Input: part model. Units: mm. Frame: model coordinates. A direction names the side the tool comes from. Coordinates: 2 decimals unless noted, no trailing zeros. Write each loop counter-clockwise with the first axis right and the second up, starting at its lowest first coordinate (ties: lowest second). Pieces come first, ordered by that corner, then holes. Notation, with made-up numbers: M 45,59 L 67,59 A29 ccw 67,85 Z; hole C 24,0 d2. An arc over 180 degrees is marked long. Write each question's results on one line, items separated by ' | '. Start each with the question number.
1. First-contact query: pin 1 (1 mm diameter, centred on y = 86, z = 6.5, fed in from -X); pin 2 (2 mm diameter, centred on x = -41.5, z = 8, fed in from +Y); pin 3 (1 mm diameter, centred on y = 25, z = 4.5, fed in from +X). Flat tips, straight axial feed; report the tip coordinate or a pass-through.
2. Section query B-B, the plane x = -20.5. Output: boundary loops of the cut face in (y, z) (3 decimals).
3. Section query C-C, the plane y = 9. Output: boundary loops of the cut face in (x, z).
4. Section query A-A, the plane z = 4.75. Output: boundary loops of the cut face in (x, y).
5. Set-up query: faces 1 (the flat face through (-98, 98, 2.54)), 2 (the flat face through (-94, 99, 10.16)), 3 (the flat face through (-139, 0, 2)). Return all of +Z, -Z, +X, -X, +Y, -Y with unobstructed straight access to the full face (end or side cutting, diameter ignored); none if empty.
6. Pull-direction query (X, two-part tool) for faces 4 (the flat face through (0, 137, 4)), 5 (the flat face through (-89, 89, 0)), 6 (the cylindrical face through (-4.45, 4.53, 1.25)); classes: +X half, -X half, draft (parallel to the pull), parting line (faces both ways), or undercut.
7. Ray query, probe 1 along Z at (x, y) = (-120.5, 67); probe 2 along Y at (x, z) = (-57.15, 1.3); probe 3 along X at (y, z) = (64.5, 3.75). Return the intervals inside material, ascending.
8. Section query D-D, the plane x = -63.5. Output: boundary loops of the cut face in (y, z), and give its area (3 significant figures).
```python
from build123d import *

# Parameters (mm, degrees)
F1_DEPTH = 2.54
F2_DEPTH = 7.62
F3_DEPTH = 2.54
F4_DEPTH = 15.24


with BuildPart() as f1:
    # F0 (on Top) → F1 (new body)
    with BuildSketch(Plane.XY):
        with BuildLine():
            Line((-6.2754395375, 0.9702363687), (-12.7, 1.9635281017))
            Line((-12.7, 1.9635281017), (-12.7, 0))
            Line((-12.7, 0), (-6.35, 0))
            ThreePointArc((-6.35, 0), (-6.3313324452, 0.4865485263), (-6.2754395375, 0.9702363687))
        make_face()
        with BuildLine():
            Line((-6.35, 0), (-2.54, 0))
            ThreePointArc((-2.54, 0), (-2.5325329781, 0.1946194105), (-2.510175815, 0.3880945475))
            Line((-2.510175815, 0.3880945475), (-6.2754395375, 0.9702363687))
            ThreePointArc((-6.2754395375, 0.9702363687), (-6.3313324452, 0.4865485263), (-6.35, 0))
        make_face()
        with BuildLine():
            ThreePointArc((-2.510175815, 0.3880945475), (-1.7960512242, 1.7960512242), (-0.3880945475, 2.510175815))
            Line((-0.3880945475, 2.510175815), (-0.9702363687, 6.2754395375))
            ThreePointArc((-0.9702363687, 6.2754395375), (-4.4901280605, 4.4901280605), (-6.2754395375, 0.9702363687))
            Line((-6.2754395375, 0.9702363687), (-2.510175815, 0.3880945475))
        make_face()
        with BuildLine():
            Line((0, 2.54), (0, 6.35))
            ThreePointArc((0, 6.35), (-0.4865485263, 6.3313324452), (-0.9702363687, 6.2754395375))
            Line((-0.9702363687, 6.2754395375), (-0.3880945475, 2.510175815))
            ThreePointArc((-0.3880945475, 2.510175815), (-0.1946194105, 2.5325329781), (0, 2.54))
        make_face()
        with BuildLine():
            Line((0, 6.35), (0, 12.7))
            Line((0, 12.7), (-1.9635281017, 12.7))
            Line((-1.9635281017, 12.7), (-0.9702363687, 6.2754395375))
            ThreePointArc((-0.9702363687, 6.2754395375), (-0.4865485263, 6.3313324452), (0, 6.35))
        make_face()
        with BuildLine():
            Line((0, 12.7), (0, 30.48))
            ThreePointArc((0, 30.48), (-2.3354329262, 30.3903957369), (-4.6571345698, 30.12210978))
            Line((-4.6571345698, 30.12210978), (-1.9635281017, 12.7))
            Line((-1.9635281017, 12.7), (0, 12.7))
        make_face()
        with BuildLine():
            Line((-12.7, 1.9635281017), (-30.12210978, 4.6571345698))
            ThreePointArc((-30.12210978, 4.6571345698), (-30.3903957369, 2.3354329262), (-30.48, 0))
            Line((-30.48, 0), (-12.7, 0))
            Line((-12.7, 0), (-12.7, 1.9635281017))
        make_face()
        with BuildLine():
            Line((-30.12210978, 4.6571345698), (-82.1429547439, 12.7))
            ThreePointArc((-82.1429547439, 12.7), (-79.6054840123, 6.5740037456), (-78.74, 0))
            Line((-78.74, 0), (-30.48, 0))
            ThreePointArc((-30.48, 0), (-30.3903957369, 2.3354329262), (-30.12210978, 4.6571345698))
        make_face()
        with BuildLine():
            Line((-12.7, 126.1370452561), (-12.7, 134.0196045361))
            ThreePointArc((-12.7, 134.0196045361), (-95.1907148833, 95.1907148833), (-134.0196045361, 12.7))
            Line((-134.0196045361, 12.7), (-126.1370452561, 12.7))
            ThreePointArc((-126.1370452561, 12.7), (-104.14, 25.4), (-82.1429547439, 12.7))
            Line((-82.1429547439, 12.7), (-57.15, 12.7))
            ThreePointArc((-57.15, 12.7), (-88.5808964237, 88.5808964237), (-12.7, 57.15))
            Line((-12.7, 57.15), (-12.7, 82.1429547439))
            ThreePointArc((-12.7, 82.1429547439), (-25.4, 104.14), (-12.7, 126.1370452561))
        make_face()
        with BuildLine():
            Line((-126.1370452561, 12.7), (-134.0196045361, 12.7))
            ThreePointArc((-134.0196045361, 12.7), (-134.4698173618, 6.3570919986), (-134.62, 0))
            Line((-134.62, 0), (-129.54, 0))
            ThreePointArc((-129.54, 0), (-128.6745159877, 6.5740037456), (-126.1370452561, 12.7))
        make_face()
        with BuildLine():
            Line((-57.15, 12.7), (-82.1429547439, 12.7))
            Line((-82.1429547439, 12.7), (-30.12210978, 4.6571345698))
            ThreePointArc((-30.12210978, 4.6571345698), (-29.1934246673, 8.7620977053), (-27.7081287712, 12.7))
            Line((-27.7081287712, 12.7), (-57.15, 12.7))
        make_face()
        with BuildLine():
            Line((-12.7, 27.7081287712), (-12.7, 57.15))
            ThreePointArc((-12.7, 57.15), (-25.7191035763, 25.7191035763), (-57.15, 12.7))
            Line((-57.15, 12.7), (-27.7081287712, 12.7))
            ThreePointArc((-27.7081287712, 12.7), (-21.5526146906, 21.5526146906), (-12.7, 27.7081287712))
        make_face()
        with BuildLine():
            Line((-4.6571345698, 30.12210978), (-12.7, 82.1429547439))
            Line((-12.7, 82.1429547439), (-12.7, 57.15))
            Line((-12.7, 57.15), (-12.7, 27.7081287712))
            ThreePointArc((-12.7, 27.7081287712), (-8.7620977053, 29.1934246673), (-4.6571345698, 30.12210978))
        make_face()
        with BuildLine():
            Line((0, 30.48), (0, 78.74))
            ThreePointArc((0, 78.74), (-6.5740037456, 79.6054840123), (-12.7, 82.1429547439))
            Line((-12.7, 82.1429547439), (-4.6571345698, 30.12210978))
            ThreePointArc((-4.6571345698, 30.12210978), (-2.3354329262, 30.3903957369), (0, 30.48))
        make_face()
        with BuildLine():
            Line((0, 129.54), (0, 134.62))
            ThreePointArc((0, 134.62), (-6.3570919986, 134.4698173618), (-12.7, 134.0196045361))
            Line((-12.7, 134.0196045361), (-12.7, 126.1370452561))
            ThreePointArc((-12.7, 126.1370452561), (-6.5740037456, 128.6745159877), (0, 129.54))
        make_face()
    extrude(amount=F1_DEPTH)

    # F0 (on Top) → F2 (join)
    with BuildSketch(Plane.XY):
        with BuildLine():
            ThreePointArc((-134.62, 0), (-134.4698173618, 6.3570919986), (-134.0196045361, 12.7))
            Line((-134.0196045361, 12.7), (-136.5707713971, 12.7))
            ThreePointArc((-136.5707713971, 12.7), (-137.0126136617, 6.3568307817), (-137.16, 0))
            Line((-137.16, 0), (-134.62, 0))
        make_face()
        with BuildLine():
            ThreePointArc((-134.0196045361, 12.7), (-95.1907148833, 95.1907148833), (-12.7, 134.0196045361))
            Line((-12.7, 134.0196045361), (-12.7, 136.5707713971))
            ThreePointArc((-12.7, 136.5707713971), (-96.9867661075, 96.9867661075), (-136.5707713971, 12.7))
            Line((-136.5707713971, 12.7), (-134.0196045361, 12.7))
        make_face()
        with BuildLine():
            ThreePointArc((-12.7, 134.0196045361), (-6.3570919986, 134.4698173618), (0, 134.62))
            Line((0, 134.62), (0, 137.16))
            ThreePointArc((0, 137.16), (-6.3568307817, 137.0126136617), (-12.7, 136.5707713971))
            Line((-12.7, 136.5707713971), (-12.7, 134.0196045361))
        make_face()
    extrude(amount=F2_DEPTH)

    # F0 (on Top) + F2_face (on face) → F3 (join)
    with BuildSketch(Plane.XY):
        with BuildLine():
            ThreePointArc((-137.16, 0), (-137.0126136617, 6.3568307817), (-136.5707713971, 12.7))
            Line((-136.5707713971, 12.7), (-141.6719012366, 12.7))
            ThreePointArc((-141.6719012366, 12.7), (-142.0979043334, 6.3563499), (-142.24, 0))
            Line((-142.24, 0), (-137.16, 0))
        make_face()
        with BuildLine():
            ThreePointArc((-136.5707713971, 12.7), (-96.9867661075, 96.9867661075), (-12.7, 136.5707713971))
            Line((-12.7, 136.5707713971), (-12.7, 141.6719012366))
            ThreePointArc((-12.7, 141.6719012366), (-100.578868556, 100.578868556), (-141.6719012366, 12.7))
            Line((-141.6719012366, 12.7), (-136.5707713971, 12.7))
        make_face()
        with BuildLine():
            ThreePointArc((-12.7, 136.5707713971), (-6.3568307817, 137.0126136617), (0, 137.16))
            Line((0, 137.16), (0, 142.24))
            ThreePointArc((0, 142.24), (-6.3563499, 142.0979043334), (-12.7, 141.6719012366))
            Line((-12.7, 141.6719012366), (-12.7, 136.5707713971))
        make_face()
    with BuildSketch(Plane(origin=(-86.5127795808, 86.5127795808, 7.62), x_dir=(1, 0, 0), z_dir=(0, 0, 1))):
        with BuildLine():
            Line((-50.6472204192, -86.5127795808), (-48.1072204192, -86.5127795808))
            ThreePointArc((-48.1072204192, -86.5127795808), (-8.6779353026, 8.6779353025), (86.5127795808, 48.1072204192))
            Line((86.5127795808, 48.1072204192), (86.5127795808, 50.6472204192))
            ThreePointArc((86.5127795808, 50.6472204192), (-10.4739865268, 10.4739865267), (-50.6472204192, -86.5127795808))
        make_face()
    extrude(amount=F3_DEPTH)

    # F0 (on Top) → F4 (join)
    with BuildSketch(Plane.XY):
        with BuildLine():
            ThreePointArc((-142.24, 0), (-142.0979043334, 6.3563499), (-141.6719012366, 12.7))
            Line((-141.6719012366, 12.7), (-144.2219067964, 12.7))
            ThreePointArc((-144.2219067964, 12.7), (-144.6404094055, 6.3561283031), (-144.78, 0))
            Line((-144.78, 0), (-142.24, 0))
        make_face()
        with BuildLine():
            ThreePointArc((-141.6719012366, 12.7), (-100.578868556, 100.578868556), (-12.7, 141.6719012366))
            Line((-12.7, 141.6719012366), (-12.7, 144.2219067964))
            ThreePointArc((-12.7, 144.2219067964), (-102.3749197802, 102.3749197802), (-144.2219067964, 12.7))
            Line((-144.2219067964, 12.7), (-141.6719012366, 12.7))
        make_face()
        with BuildLine():
            ThreePointArc((-12.7, 141.6719012366), (-6.3563499, 142.0979043334), (0, 142.24))
            Line((0, 142.24), (0, 144.78))
            ThreePointArc((0, 144.78), (-6.3561283031, 144.6404094055), (-12.7, 144.2219067964))
            Line((-12.7, 144.2219067964), (-12.7, 141.6719012366))
        make_face()
    extrude(amount=F4_DEPTH)


solid = f1.part
```
Answer:
1) pin 1: x = -116.84 | pin 2: y = 139 | pin 3: x = -132.18
2) outline: M 0,0 L 3.169,0 L 3.169,2.54 L 0,2.54 Z; M 22.556,0 L 31.999,0 L 31.999,2.54 L 22.556,2.54 Z; M 82.301,0 L 89.143,0 L 89.143,2.54 L 82.301,2.54 Z; M 119.137,0 L 143.321,0 L 143.321,15.24 L 140.755,15.24 L 140.755,2.54 L 135.619,2.54 L 135.619,10.16 L 133.05,10.16 L 133.05,2.54 L 119.137,2.54 Z
3) outline: M -144.5,0 L -127.89,0 L -127.89,2.54 L -134.32,2.54 L -134.32,10.16 L -136.86,10.16 L -136.86,2.54 L -141.95,2.54 L -141.95,15.24 L -144.5,15.24 Z; M -80.39,0 L -29.12,0 L -29.12,2.54 L -80.39,2.54 Z; M -1.39,0 L 0,0 L 0,2.54 L -1.39,2.54 Z
4) outline: M -144.78,0 L -142.24,0 A142.24 cw 0,142.24 L 0,144.78 A144.78 ccw Z; M -137.16,0 L -134.62,0 A134.62 cw 0,134.62 L 0,137.16 A137.16 ccw Z
5) face 1: +Z | face 2: +Z, +X, -Y | face 3: +Z, -Z, +X, -X, -Y
6) face 4: +X half | face 5: draft | face 6: undercut
7) probe 1: 0 to 2.54 | probe 2: 0 to 12.7, 101.6 to 133.02 | probe 3: -129.62 to -126.78, -121.05 to -118.16
8) outline: M 0,0 L 13.16,0 L 13.16,2.54 L 0,2.54 Z; M 101.14,0 L 130.11,0 L 130.11,15.24 L 127.28,15.24 L 127.28,2.54 L 121.58,2.54 L 121.58,10.16 L 118.7,10.16 L 118.7,2.54 L 101.14,2.54 Z | area: 165 mm^2
